from build123d import *

# Parameters (mm, degrees)
FILLET1_R = 3.175
FILLET4_R = 1.524


with BuildPart() as part:
    # Sketch1 → Revolve1 (revolve)
    with BuildSketch(Plane(origin=(0, 0, 0), x_dir=(0, 0, -1), z_dir=(1, 0, 0)), mode=Mode.PRIVATE) as revolve1_sk:
        Polygon((-1.651, 0), (-1.651, 7.9375), (-6.35, 7.9375), (-6.35, 6.35), (-4.7625, 6.35), (-4.7625, 0), align=None)
    revolve(revolve1_sk.sketch.rotate(Axis((0, 0, 0), (0, 1, 0)), 180), axis=Axis((0, 0, 0), (0, 1, 0)))

    # Fillet1
    fillet1_edges = [part.edges().sort_by_distance(p)[0] for p in [
        (0, 7.9375, 1.651),
    ]]
    fillet(fillet1_edges, radius=FILLET1_R)

    # Fillet4
    fillet4_edges = [part.edges().sort_by_distance(p)[0] for p in [
        (0, 0, 4.7625),
        (0, 0, 1.651),
    ]]
    fillet(fillet4_edges, radius=FILLET4_R)


solid = part.part
Model file for the job. Use its own axes, mm. A direction names the side the tool comes from. Coordinates: 2 decimals unless noted, no trailing zeros. Write each loop counter-clockwise with the first axis right and the second up, starting at its lowest first coordinate (ties: lowest second). Pieces come first, ordered by that corner, then holes. Notation, with made-up numbers: (87.5, 84.5) - (119.5, 84.5) arc R14 cw to (119.5, 98.5) - close; hole circle Ø11 at (61.25, 7). An arc over 180 degrees is marked (long way). Write each question's results on one line, items separated by ' | '. Start each with the question number.
1) Cut at D-D (z = 5.5). Write the cut outline in (x, y).
2) Mould opens along Z. For faces 1 (the face through (-5, 6.35, -1)), 2 (the face through (-0.496, 3.166, -1.575)), 3 (the face through (5.634, 7.133, -2.93)) say: pulls with the +Z half, pulls with the -Z half, needs draft (parallel to the pull), parting line crosses it, or undercut.
3) Probe line 1 along X through (y, z) = (3.6, 0); line 2 along Y through (x, z) = (3, 4.75); line 3 along X through (y, z) = (5.25, -1.25). List the from-to ranges inside material, lowest first. Write a range as from..to.
4) Cut at C-C (y = 2.25). Write the cut outline in (x, z) (1 decimal), then the cut area to 3 significant figures.
5) 3-axis set-ups, long thin cutter, end or side, ignore diameter. For faces 4 (the face through (-5, 7.938, -1)), 5 (the face through (4.65, 3.9, 1.03)): which of +Z, -Z, +X, -X, +Y, -Y reach the whole face in a straight line?
6) Flat gauge pins, fed straight in: P1, Ø2, axis at y = 6, z = -0.5, coming from the +X side; P2, Ø4, axis at y = 3.5, z = 4, coming from the +X side; P3, Ø1, axis at x = -4.5, z = -4.5, coming from the -Y side; P4, Ø1.5, axis at y = 3.5, z = -1.5, coming from the -X side. Where does each tip first touch, or does it go through?
Returned:
1) outline: (-3.17, 6.35) - (3.17, 6.35) - (3.17, 7.94) - (-3.17, 7.94) - close
2) face 1: needs draft | face 2: undercut | face 3: parting line crosses it
3) line 1: -4.76..-1.65, 1.65..4.76 | line 2: 6.35..7.94 | line 3: -4.6..-1.14, 1.14..4.6
4) outline: circle Ø9.5 at (0, 0); hole circle Ø3.3 at (0, 0) | area: 62.7 mm^2
5) face 4: +Z, -Z, +X, -X, +Y | face 5: -Y
6) P1: x = 6.35 | P2: x = 4.32 | P3: y = 6.35 | P4: x = -4.7
